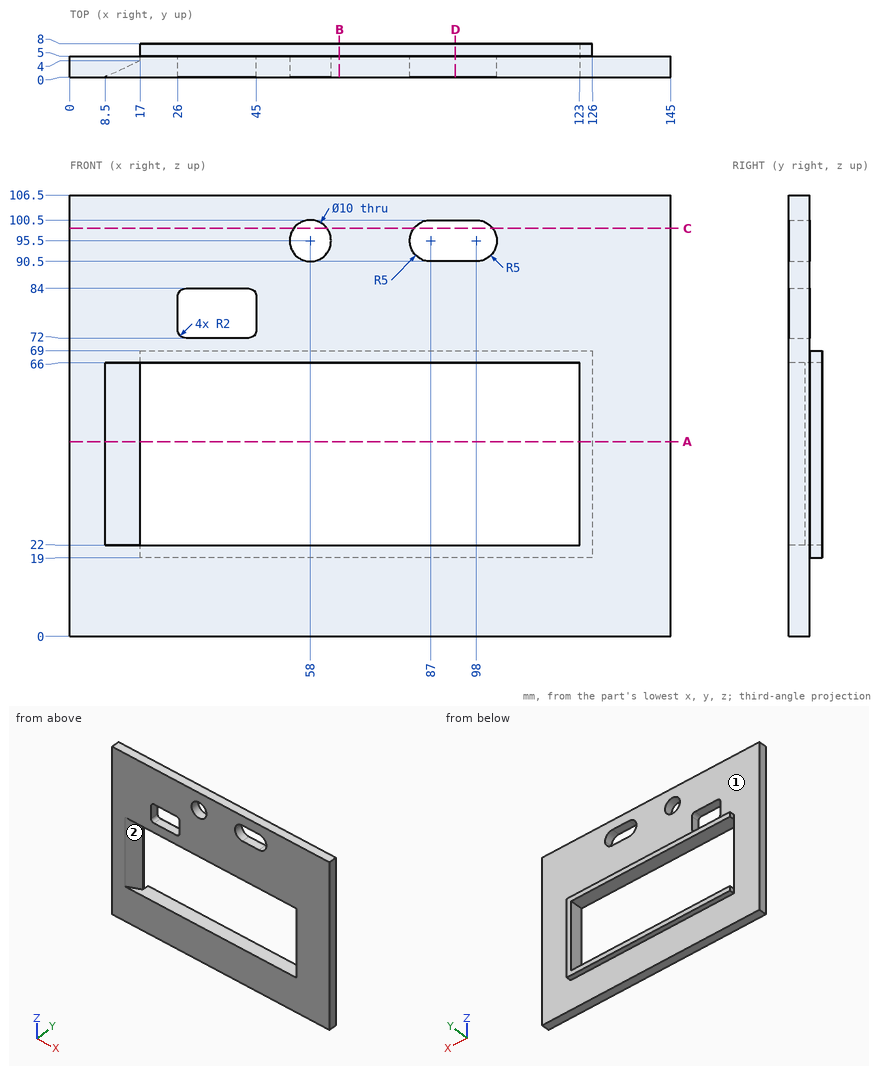
Input: dimensioned drawing with shaded views. Units: mm. Origin: part minimum x, y, z. Give positions to 0.01 mm unless a question says otherwise; leave off trailing zeros. Loops run counter-clockwise (first coordinate to the right, second up) from the corner with the lowest first, then second, coordinate; pieces in that order, holes last. Notation, with made-up numbers: (39, 63.5) - (56, 63.5) arc R22 ccw to (56, 90.5) - close; hole circle Ø6 at (68.25, -0.5). An arc over 180 degrees is marked (long way). Answer as CSV lines item,"result". Start each with the question number.
(1) Section query D-D (x = 93). Output: boundary loops of the cut face in (y, z), and give its area (4 significant figures).
(2) Section query B-B (x = 65). Output: boundary loops of the cut face in (y, z), and give its area (4 significant figures).
(3) Section query C-C (z = 98.5). Output: boundary loops of the cut face in (x, y), and give its area (3 significant figures).
(4) Mould query, pull axis Z, two halves, no side actions, for the marked faces 1 and 2. Classes: +Z half, -Z half, draft (parallel to the pull), parting line (faces both ways), or undercut.
(5) Section query A-A (z = 47). Output: boundary loops of the cut face in (x, y), and give its area (3 significant figures).
(6) Ray query, line 1 along Z through (x, y) = (58, 2.3); line 2 along Z through (x, y) = (102.5, 7.5); line 3 along Z through (x, y) = (65, 1.5). Return the intervals inside material, ascending. Write a range as [from, to].
(7) Pin query (flat end, axial travel): P1, Ø3.5, axis at y = 6.5, z = 67, coming from the -X side; P2, Ø16, axis at x = 58, z = 95.5, coming from the +Y side; P3, Ø3.5, axis at x = 84.5, y = 7, coming from the +Z side. Return the tip coordinate at first contact, or that it passes through.
Worked answers:
1,outline,"(0, 0) - (5, 0) - (5, 19) - (8, 19) - (8, 22) - (0, 22) - close; (0, 66) - (8, 66) - (8, 69) - (5, 69) - (5, 90.5) - (0, 90.5) - close; (0, 100.5) - (5, 100.5) - (5, 106.5) - (0, 106.5) - close"
1,area,"280.5 mm^2"
2,outline,"(0, 0) - (5, 0) - (5, 19) - (8, 19) - (8, 22) - (0, 22) - close; (0, 66) - (8, 66) - (8, 69) - (5, 69) - (5, 106.5) - (0, 106.5) - close"
2,area,"330.5 mm^2"
3,outline,"(0, 0) - (54, 0) - (54, 5) - (0, 5) - close; (62, 0) - (83, 0) - (83, 5) - (62, 5) - close; (102, 0) - (145, 0) - (145, 5) - (102, 5) - close"
3,area,"590 mm^2"
4,face 1,"draft"
4,face 2,"undercut"
5,outline,"(0, 0) - (8.5, 0) - (17, 4) - (17, 5) - (0, 5) - close; (123, 0) - (145, 0) - (145, 5) - (126, 5) - (126, 8) - (123, 8) - close"
5,area,"187 mm^2"
6,line 1,"z = [0, 22], [66, 90.5], [100.5, 106.5]"
6,line 2,"z = [19, 22], [66, 69]"
6,line 3,"z = [0, 22], [66, 106.5]"
7,P1,"stops at x = 0"
7,P2,"stops at y = 5"
7,P3,"stops at z = 69"
